Input: part model. Units: mm. Frame: model coordinates. Face numbers are marked on the shaded views. Give positions to 0.01 mm unless a question says otherwise; leave off trailing zeros. Loops run counter-clockwise (first coordinate to the right, second up) from the corner with the lowest first, then second, coordinate; pieces in that order, holes last. Notation, with made-up numbers: (-33.5, 83) - (-25.5, 83) arc R34 cw to (-25.5, 117) - close; hole circle Ø8 at (61, -33.75). An arc over 180 degrees is marked (long way). Answer as a JSON object with one key per item and string values. Group by question number.
(1) Section query B-B (y = 0). Return loops of the section in (x, z).
(2) Section query D-D (z = -15). Return loops of the section in (x, y).
(3) Material intervals for L1, parallel to Y at x = 0, z = 7; L2, parallel to Y at x = 0, z = -3; L3, parallel to Z at x = -1.75, y = -3, sorted ascending.
(4) Mould query, pull axis X, two halves, no side actions, for the marked faces 1, 2 and 3. Classes: +X half, -X half, draft (parallel to the pull), parting line (faces both ways), or undercut.
(5) Section query C-C (z = 0). Return loops of the section in (x, y).
(6) Pin query (flat end, axial travel): P1, Ø5, axis at x = 0, y = -25, coming from the -Z side; P2, Ø16, axis at y = 0, z = 0, coming from the -X side. Return the tip coordinate at first contact, or that it passes through.
(7) Section query A-A (x = 0). Return loops of the section in (y, z), plus the area to 3 significant figures.
```python
from build123d import *

# Parameters (mm, degrees)
CROQUIS1_W                    = 35
CROQUIS1_H                    = 70
CROQUIS1_R                    = 5
SALIENTE_EXTRUIR1_DEPTH       = 6.35
DI_METRO_DE_TALADRO_5_0_5_1_D = 8


with BuildPart() as part:
    # Croquis1 → Saliente-Extruir1 (new, symmetric)
    with BuildSketch(Plane(origin=(0, 0, 0), x_dir=(0, 0, -1), z_dir=(1, 0, 0))):
        Rectangle(CROQUIS1_W, CROQUIS1_H)
        Circle(CROQUIS1_R, mode=Mode.SUBTRACT)
    extrude(amount=SALIENTE_EXTRUIR1_DEPTH, both=True)

    # Diámetro de taladro Ø5.0 (5)1 (through all)
    with Locations(Plane.XY.offset(17.5)):
        with Locations((0, 25), (0, -25)):
            Hole(DI_METRO_DE_TALADRO_5_0_5_1_D / 2)


solid = part.part
```
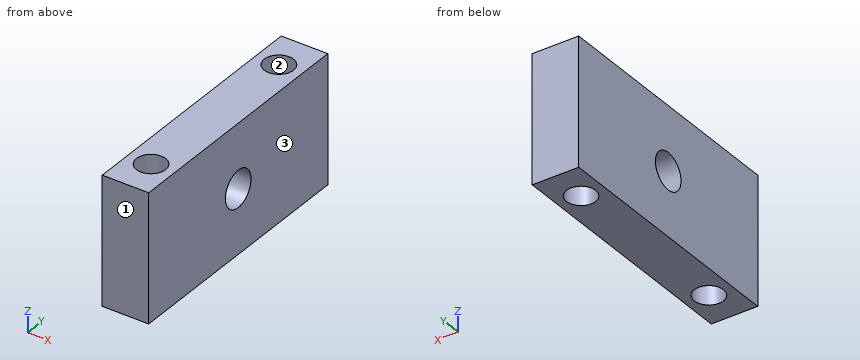
Recorded:
{
 "1": {"outline": "(-6.35, -17.5) - (6.35, -17.5) - (6.35, -5) - (-6.35, -5) - close; (-6.35, 5) - (6.35, 5) - (6.35, 17.5) - (-6.35, 17.5) - close"},
 "2": {"outline": "(-6.35, -35) - (6.35, -35) - (6.35, 35) - (-6.35, 35) - close; hole circle Ø8 at (0, -25); hole circle Ø8 at (0, 25)"},
 "3": {"L1": "y = -35 to -29, -21 to 21, 29 to 35", "L2": "y = -35 to -29, -21 to -4, 4 to 21, 29 to 35", "L3": "z = -17.5 to -4, 4 to 17.5"},
 "4": {"face 1": "draft", "face 2": "undercut", "face 3": "+X half"},
 "5": {"outline": "(-6.35, -35) - (6.35, -35) - (6.35, -5) - (-6.35, -5) - close; (-6.35, 5) - (6.35, 5) - (6.35, 35) - (-6.35, 35) - close; hole circle Ø8 at (0, -25); hole circle Ø8 at (0, 25)"},
 "6": {"P1": "passes through", "P2": "stops at x = -6.35"},
 "7": {"outline": "(-35, -17.5) - (-29, -17.5) - (-29, 17.5) - (-35, 17.5) - close; (-21, -17.5) - (21, -17.5) - (21, 17.5) - (-21, 17.5) - close; (29, -17.5) - (35, -17.5) - (35, 17.5) - (29, 17.5) - close; hole circle Ø10 at (0, 0)", "area": "1,810 mm^2"}
}
